Verification items for this drawing (mm, ordinates from the low corner). A direction names the side the tool comes from. Coordinates: 2 decimals unless noted, no trailing zeros. Order: outer loops, then holes, each group sorted by start corner. A loop starts at its lowest first (then second) coordinate and runs counter-clockwise, first axis right, second up. Notation, with made-up numbers: M 84,85.25 L 116,85.25 A29 ccw 116,121.25 Z; hole C -10.75,0 d1. An arc over 180 degrees is marked long. Return JSON: item names as keys, results as strings. Group by question number.
1. Set-up check for the marked faces 4, 5 and 6: record each of +Z, -Z, +X, -X, +Y, -Y from which the full face is reachable in a straight line by a thin tool's end or side.
2. Section check B-B, the plane z = 2.35. Record the cut outline in (x, y) (1 decimal), plus the area to 3 significant figures.
3. Section check C-C, the plane y = 15.25. Record the cut outline in (x, z), plus the area to 3 significant figures.
4. Mould release check, pull along X, two halves, no side actions. Record for the marked faces 1, 2 and 3: +X half, -X half, draft (parallel to the pull), parting line (faces both ways), or undercut.
5. Section check A-A, the plane x = 9.25. Record the cut outline in (y, z) (1 decimal), plus the area to 3 significant figures.
6. Gauge pin test, flat ends, axial feed: pin 1 (1.6 mm diameter, centred on y = 12.5, z = 2, fed in from -X); pin 2 (0.8 mm diameter, centred on x = 9.5, z = 2.5, fed in from -Y) (1 decimal); pin 3 (2 mm diameter, centred on x = 9.65, y = 2.82, fed in from -Z); pin 4 (0.8 mm diameter, centred on x = 8.5, z = 2.5, fed in from +Y). Record the tip position at first contact, or that the pin passes through.
7. Material ranges on line 1 along Y through (x, z) = (9.75, 0.75) (1 decimal); line 2 along Z through (x, y) = (4, 16); line 3 along Y through (x, z) = (8, 2.6) (1 decimal), recorded low to high.
8. Section check D-D, the plane x = 7.5. Record the cut outline in (y, z) (1 decimal), plus the area to 3 significant figures.
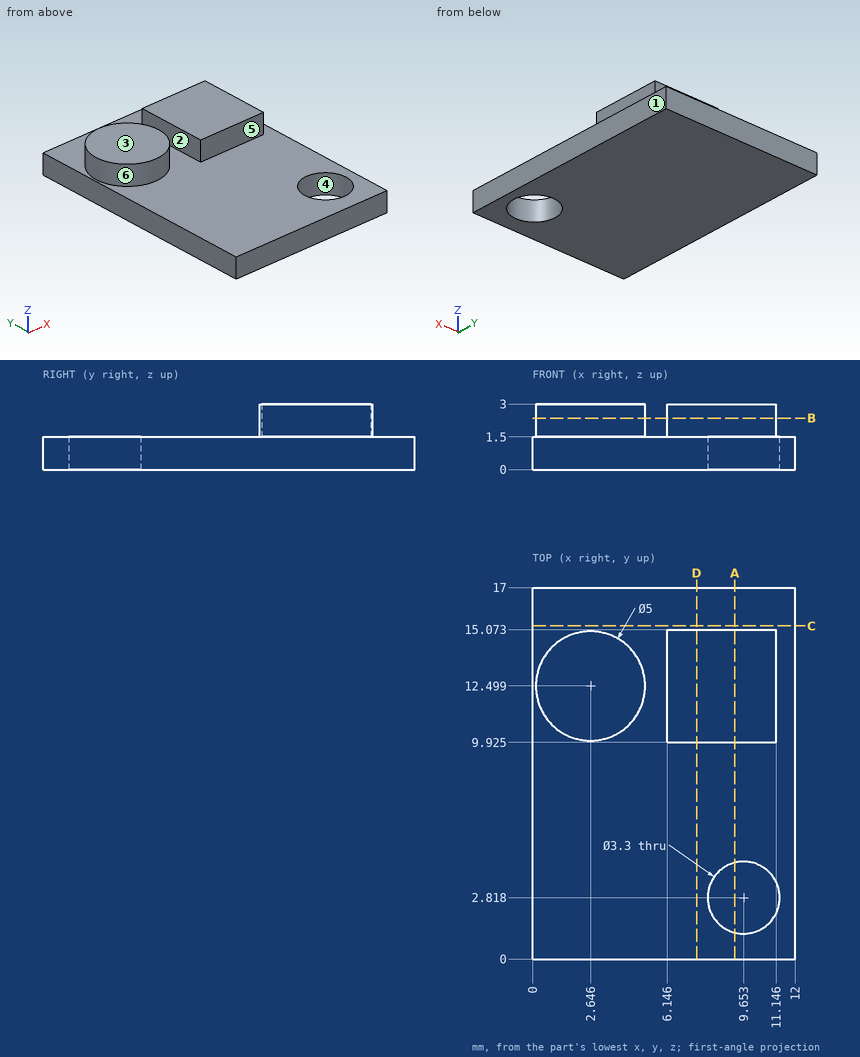
Answers follow:
{
 "1": {"face 4": "+Z, -Z", "face 5": "+Z, +X, -X, -Y", "face 6": "+Z"},
 "2": {"outline": "C 2.6,12.5 d5; M 6.1,9.9 L 11.1,9.9 L 11.1,15.1 L 6.1,15.1 Z", "area": "45.4 mm^2"},
 "3": {"outline": "M 0,0 L 12,0 L 12,1.5 L 0,1.5 Z", "area": "18.0 mm^2"},
 "4": {"face 1": "+X half", "face 2": "undercut", "face 3": "draft"},
 "5": {"outline": "M 0,0 L 1.2,0 L 1.2,1.5 L 0,1.5 Z; M 4.4,0 L 17,0 L 17,1.5 L 15.1,1.5 L 15.1,3 L 9.9,3 L 9.9,1.5 L 4.4,1.5 Z", "area": "28.4 mm^2"},
 "6": {"pin 1": "x = 0", "pin 2": "y = 9.9", "pin 3": "through", "pin 4": "y = 15.07"},
 "7": {"line 1": "0 to 1.2, 4.5 to 17", "line 2": "0 to 1.5", "line 3": "9.9 to 15.1"},
 "8": {"outline": "M 0,0 L 17,0 L 17,1.5 L 15.1,1.5 L 15.1,3 L 9.9,3 L 9.9,1.5 L 0,1.5 Z", "area": "33.2 mm^2"}
}
